Here's how the part is built. I have some questions about the finished solid (model axes, mm). A direction names the side the tool comes from. Give positions to 0.01 mm unless a question says otherwise; leave off trailing zeros. Loops run counter-clockwise (first coordinate to the right, second up) from the corner with the lowest first, then second, coordinate; pieces in that order, holes last. Notation, with made-up numbers: (-7, 14) - (11, 14) arc R31 cw to (11, 40) - close; hole circle Ø7 at (55.25, 74). An arc over 180 degrees is marked (long way). One line per item, written item: value. Start each with the question number.
Autodesk Inventor part; units mm, degrees
ref_plane "YZ Plane" through (0, 0, 0) normal (1, 0, 0) x (0, 1, 0)
ref_plane "XZ Plane" through (0, 0, 0) normal (0, 1, 0) x (-1, 0, 0)
ref_plane "XY Plane" through (0, 0, 0) normal (0, 0, 1) x (1, 0, 0)
sketch "Sketch1" plane through (0, 0, 0) normal (1, 0, 0) x (0, 1, 0)
  circle A0 centre (0, 0) radius 9.5
  line L0 (-30, -110.28) -> (30, -110.28)
  line L1 (30, -110.28) -> (30, 110.28)
  line L2 (30, 110.28) -> (-30, 110.28)
  line L3 (-30, 110.28) -> (-30, -110.28)
  line L4 (-30, -110.28) -> (30, 110.28) construction
  line L5 (30, -110.28) -> (-30, 110.28) construction
  line L6 (30, -110.28) -> (-30, -110.28)
  line L7 (-30, -110.28) -> (-30, -339.72)
  line L8 (-30, -339.72) -> (30, -339.72)
  line L9 (30, -339.72) -> (30, -110.28)
  circle A1 centre (0, -311.7) radius 3.25
  dimension "d0" = 19
  dimension "d1" = 60
  dimension "d2" = 220.56
  dimension "d5" = 60
  dimension "d6" = 229.44
  dimension "d8" = 6.5
  dimension "d9" = 28.02
  dimension "d10" = 30
extrude "Extrusion1" add sketch "Sketch1" along normal blind 7 contours L3 L2 L1 L0 | L0 L9 L8 L7 | A1
sketch "Sketch2" plane through (7, 0, 0) normal (-1, 0, 0) x (0, 0, 1)
  circle A0 centre (0, 0) radius 11
  dimension "d11" = 22
extrude "Extrusion2" cut sketch "Sketch2" along normal blind 1.2
sketch "Sketch3" plane through (7, 0, 0) normal (1, 0, 0) x (0, 0, -1)
  circle A0 centre (-98.28, 16.75) radius 2.75
  circle A1 centre (-98.28, -16.75) radius 2.75
  circle A2 centre (324.72, 16.75) radius 2.75
  circle A3 centre (324.72, -16.75) radius 2.75
  line L0 (-110.28, -30) -> (339.72, -30)
  line L1 (339.72, 30) -> (-110.28, 30)
  line L2 (339.72, -30) -> (339.72, 30)
  line L3 (-110.28, 30) -> (-110.28, -30)
  line L4 (339.72, -30) -> (309.72, -30)
  line L5 (309.72, -30) -> (309.72, 30)
  line L6 (309.72, 30) -> (339.72, 30)
  line L7 (339.72, 30) -> (339.72, -30)
  line L8 (-110.28, -30) -> (-80.28, -30)
  line L9 (-80.28, -30) -> (-80.28, 30)
  line L10 (-80.28, 30) -> (-110.28, 30)
  line L11 (-110.28, 30) -> (-110.28, -30)
  circle A4 centre (-35.28, 0) radius 20
  line L12 (-60.28, -20) -> (-10.28, -20)
  line L13 (-10.28, -20) -> (-10.28, 20)
  line L14 (-10.28, 20) -> (-60.28, 20)
  line L15 (-60.28, 20) -> (-60.28, -20)
  line L16 (-60.28, -20) -> (-10.28, 20) construction
  line L17 (-10.28, -20) -> (-60.28, 20) construction
  circle A5 centre (-60.28, 20) radius 2.75
  circle A6 centre (-10.28, 20) radius 2.75
  circle A7 centre (-60.28, -20) radius 2.75
  circle A8 centre (-10.28, -20) radius 2.75
  circle A9 centre (-10.28, 20) radius 2.75
  circle A10 centre (-10.28, -20) radius 2.75
  circle A11 centre (14.72, 0) radius 20
  circle A12 centre (39.72, 20) radius 2.75
  circle A13 centre (39.72, -20) radius 2.75
  circle A14 centre (39.72, 20) radius 2.75
  circle A15 centre (39.72, -20) radius 2.75
  circle A16 centre (64.72, 0) radius 20
  circle A17 centre (89.72, 20) radius 2.75
  circle A18 centre (89.72, -20) radius 2.75
  circle A19 centre (89.72, 20) radius 2.75
  circle A20 centre (89.72, -20) radius 2.75
  circle A21 centre (114.72, 0) radius 20
  circle A22 centre (139.72, 20) radius 2.75
  circle A23 centre (139.72, -20) radius 2.75
  circle A24 centre (139.72, 20) radius 2.75
  circle A25 centre (139.72, -20) radius 2.75
  circle A26 centre (164.72, 0) radius 20
  circle A27 centre (189.72, 20) radius 2.75
  circle A28 centre (189.72, -20) radius 2.75
  circle A29 centre (189.72, 20) radius 2.75
  circle A30 centre (189.72, -20) radius 2.75
  circle A31 centre (214.72, 0) radius 20
  circle A32 centre (239.72, 20) radius 2.75
  circle A33 centre (239.72, -20) radius 2.75
  circle A34 centre (239.72, 20) radius 2.75
  circle A35 centre (239.72, -20) radius 2.75
  circle A36 centre (264.72, 0) radius 20
  circle A37 centre (289.72, 20) radius 2.75
  circle A38 centre (289.72, -20) radius 2.75
  circle A39 centre (289.72, 20) radius 2.75
  circle A40 centre (289.72, -20) radius 2.75
  circle A41 centre (314.72, 0) radius 20
  circle A42 centre (339.72, 20) radius 2.75
  circle A43 centre (339.72, -20) radius 2.75
  circle A44 centre (339.72, 20) radius 2.75
  circle A45 centre (339.72, -20) radius 2.75
  circle A46 centre (364.72, 0) radius 20
  circle A47 centre (389.72, 20) radius 2.75
  circle A48 centre (389.72, -20) radius 2.75
  circle A49 centre (389.72, 20) radius 2.75
  circle A50 centre (389.72, -20) radius 2.75
  circle A51 centre (414.72, 0) radius 20
  circle A52 centre (439.72, 20) radius 2.75
  circle A53 centre (439.72, -20) radius 2.75
  point P0 (0, 0)
  dimension "d14" = 5.5
  dimension "d15" = 5.5
  dimension "d16" = 5.5
  dimension "d17" = 5.5
  dimension "d18" = 13.25
  dimension "d19" = 13.25
  dimension "d20" = 15
  dimension "d21" = 15
  dimension "d22" = 13.25
  dimension "d23" = 12
  dimension "d24" = 12
  dimension "d25" = 13.25
  dimension "d26" = 30
  dimension "d27" = 30
  dimension "d28" = 60
  dimension "d29" = 40
  dimension "d30" = 50
  dimension "d31" = 40
  dimension "d32" = 75
  dimension "d33" = 10
  dimension "d34" = 5.5
  dimension "d35" = 5.5
  dimension "d36" = 5.5
  dimension "d37" = 5.5
  dimension "d40" = 50
extrude "Extrusion3" cut sketch "Sketch3" against normal blind 10 contours A0 | A1 | A2 A41 | A41 A2 | A41 A3 | A3 A41 | A4 | A6 L13 L14 | L14 L13 A6 | A5 L15 L14 | L14 L15 A5 | A7 L15 L12 | L12 L15 A7 | A8 L13 L12 | L12 L13 A8 | A12 | A13 | A16 | A17 | A18 | A21 | A22 | A23 | A26 | A27 | A28 | A31 | A32 | A33 | A36 | A37 | A38
properties part number "Outer Plate Module" material "Aluminum 6061"
(1) If we mould it in two halves opening along Z, with no side actions, what happens to faces 1 (the face through (3, 0, -339.72)), 2 (the face through (3, 30, -118)), 3 (the face through (3.55, 0.88, -94.74)), 4 (the face through (3, 0, 110.28))? For each: pulls with the +Z half, pulls with the -Z half, needs draft (parallel to the pull), parting line crosses it, or undercut.
(2) For faces 5 (the face through (3, -30, -112)), 6 (the face through (5.8, 0, -10)), which set-ups out of +Z, -Z, +X, -X, +Y, -Y let a thin tool reach every point of the face, with its end or its side?
(3) Please list where these lines run through material, in increasing order: probe 1 along Y at (x, z) = (5, -189.72); probe 2 along Y at (x, z) = (2.5, -324.72); probe 3 along Y at (x, z) = (5.75, -214.72). Write a range as from..to.
(4) If we section it at B-B on z = -280: List the corners of the cut face in (x, y) for me, plus the area to 3 significant figures.
(5) If we section it at A-A on x = 3.75: Give the number of separate pieces and of enclosed holes in the cut face, plus the area to 3 significant figures.
Found:
1. face 1: pulls with the -Z half
1. face 2: needs draft
1. face 3: undercut
1. face 4: pulls with the +Z half
2. face 5: +Z, -Z, +X, -X, -Y
2. face 6: +X
3. probe 1: -30..-22.75, -17.25..17.25, 22.75..30
3. probe 2: -30..-19.5, -14..14, 19.5..30
3. probe 3: -30..-20, 20..30
4. outline: (0, -30) - (7, -30) - (7, -12.9) - (0, -12.9) - close; (0, 12.9) - (7, 12.9) - (7, 30) - (0, 30) - close
4. area: 239 mm^2
5. separate pieces: 1
5. enclosed holes: 27
5. area: 18,700 mm^2
